For this review, take the finished solid that the model builds, in its own axes (mm). Face numbers are marked on the shaded views. A direction names the side the tool comes from. Give positions to 0.01 mm unless a question says otherwise; leave off trailing zeros. Loops run counter-clockwise (first coordinate to the right, second up) from the corner with the lowest first, then second, coordinate; pieces in that order, holes last. Notation, with made-up numbers: (0.25, 74.25) - (26.25, 74.25) arc R17 cw to (26.25, 106.25) - close; hole circle Ø7 at (29, -27). An arc over 180 degrees is marked (long way). Put each result on its own line as item: value.
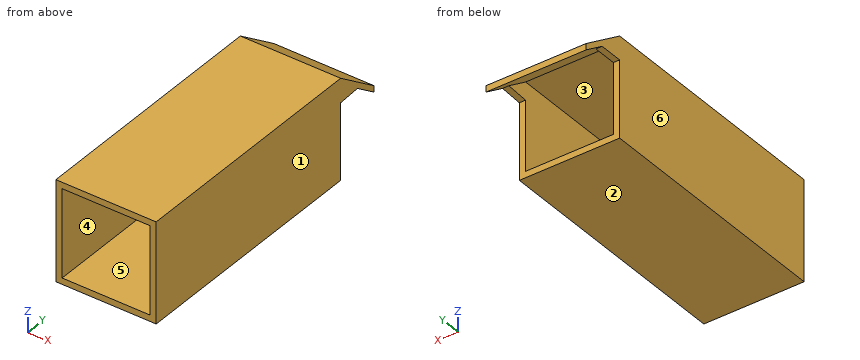
from build123d import *

# Parameters (mm, degrees)
F0_W     = 40
F0_H     = 40
F0_W_2   = 35
F0_H_2   = 35
F1_DEPTH = 100
F3_DEPTH = 40
F5_DEPTH = 2.5
F7_DEPTH = 2.5


with BuildPart() as f1:
    # F0 (on Front) → F1 (new body)
    with BuildSketch(Plane.XZ):
        with Locations((-44.507358, -17.5)):
            Rectangle(F0_W, F0_H)
        with Locations((-44.507358, -17.5)):
            Rectangle(F0_W_2, F0_H_2, mode=Mode.SUBTRACT)
    extrude(amount=F1_DEPTH)

    # F2 (on face) → F3 (join)
    with BuildSketch(Plane(origin=(-64.507358, 0, 0), x_dir=(0, -1, 0), z_dir=(-1, 0, 0))):
        Polygon((0, 0), (0, 2.5), (-18.149041, -10.649037), (-18.149041, -13.149037), align=None)
    extrude(amount=-F3_DEPTH)

    # F4 (on face) → F5 (join)
    with BuildSketch(Plane(origin=(-64.507358, 0, 0), x_dir=(0, -1, 0), z_dir=(-1, 0, 0))):
        Polygon((0, 0), (-9.484176, -6.871315), (0, -6.871315), align=None)
    extrude(amount=-F5_DEPTH)

    # F6 (on face) → F7 (join)
    with BuildSketch(Plane.YZ.offset(-24.507358)):
        Polygon((9.07452, -6.574518), (0, 0), (0, -7.108711), align=None)
    extrude(amount=-F7_DEPTH)


solid = f1.part
1) Take a section at B-B on y = -59. State the section outline as (x, z) points, and give its area (3 significant figures).
Geometry check:
outline: (-64.51, -37.5) - (-24.51, -37.5) - (-24.51, 2.5) - (-64.51, 2.5) - close; hole (-62.01, -35) - (-27.01, -35) - (-27.01, 0) - (-62.01, 0) - close
area: 375 mm²
2) For the marked faces 4, 5 and 6, list the 3-axis set-ups (+Z, -Z, +X, -X, +Y, -Y) from which the entire face can be reached by the end or side of a thin tool; tool diameter is ignored.
Geometry check:
face 4: -Y
face 5: +Y, -Y
face 6: +Z, -Z, -X, +Y, -Y
3) Draft analysis for pull direction X (two halves, no side actions). For the marked faces 1, 2 and 3, state which applies: pulls with the +X half, pulls with the -X half, needs draft (parallel to the pull), parting line crosses it, or undercut.
Geometry check:
face 1: pulls with the +X half
face 2: needs draft
face 3: undercut
4) Insertion check: pin 1 Ø8 at (x, z) = (-34.5, -7.5) entering from -Y; pin 2 Ø8 at (x, z) = (-44, -27.5) entering from +Y; pin 3 Ø6 at (x, z) = (-54, -5.5) entering from +Y; pin 4 Ø1.2 at (x, y) = (-62.5, 2.5) entering from -Z. Each pin has a flat end and moves straight along its axis. Give the tip position at first contact, or say it passes through.
Geometry check:
pin 1: stops at y = 4.83
pin 2: passes through
pin 3: stops at y = 15.18
pin 4: stops at z = -6.87
5) Take a section at A-A on x = -48.5. State the section outline as (y, z) points.
Geometry check:
outline: (-100, -37.5) - (0, -37.5) - (0, -35) - (-100, -35) - close; (-100, 0) - (0, 0) - (18.15, -13.15) - (18.15, -10.65) - (0, 2.5) - (-100, 2.5) - close
6) Wall thickness on line 1 (Z direction, x = -34, y = -93); line 2 (X direction, y = -22, z = -4); line 3 (Y direction, x = -35.5, z = -1): over which ranges is each line inside the solid? List them lowest first.
Geometry check:
line 1: z = -37.5 to -35, 0 to 2.5
line 2: x = -64.51 to -62.01, -27.01 to -24.51
line 3: y = 1.38 to 4.83
7) Take a section at D-D on z = -9.5. State the section outline as (x, y) points.
Geometry check:
outline: (-64.51, -100) - (-62.01, -100) - (-62.01, 0) - (-64.51, 0) - close; (-64.51, 13.11) - (-24.51, 13.11) - (-24.51, 16.56) - (-64.51, 16.56) - close; (-27.01, -100) - (-24.51, -100) - (-24.51, 0) - (-27.01, 0) - close
8) Take a section at C-C on z = -32.5. State the section outline as (x, y) points.
Geometry check:
outline: (-64.51, -100) - (-62.01, -100) - (-62.01, 0) - (-64.51, 0) - close; (-27.01, -100) - (-24.51, -100) - (-24.51, 0) - (-27.01, 0) - close
